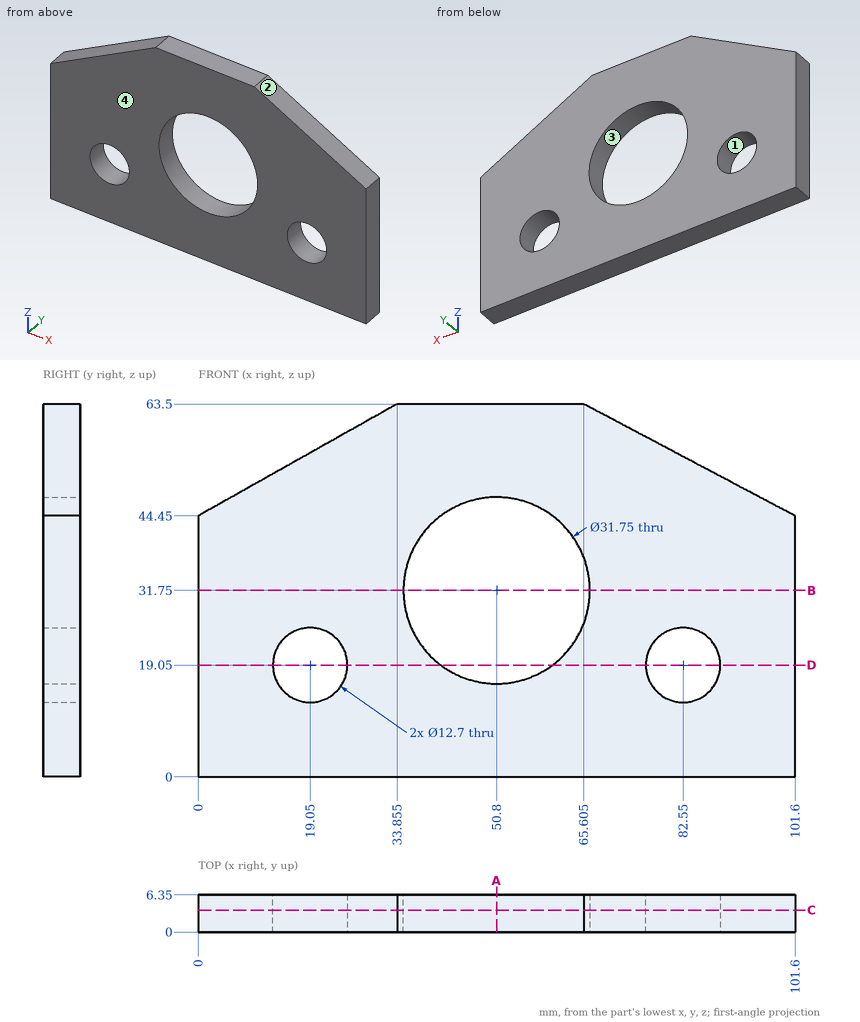
Verification items for this drawing (mm, ordinates from the low corner). Round coordinates to 2 decimals unless told otherwise and drop trailing zeros. Loops run counter-clockwise (first coordinate to the right, second up) from the corner with the lowest first, then second, coordinate; pieces in that order, holes last. Notation, with made-up numbers: (-34, 42) -> (-20, 42) arc R16 cw to (-20, 57) -> close; hole circle Ø4 at (79.25, 24). An arc over 180 degrees is marked (long way). Answer in a Markdown table with one row per item.
Q1. Sectioned sample at D-D on z = 19.05. Enter the section's corners in (x, y) (3 decimals), then the cut area to 3 significant figures.
Data:
| item | result |
|---|---|
| outline | (0, 0) -> (12.7, 0) -> (12.7, 6.35) -> (0, 6.35) -> close; (25.4, 0) -> (41.275, 0) -> (41.275, 6.35) -> (25.4, 6.35) -> close; (60.325, 0) -> (76.2, 0) -> (76.2, 6.35) -> (60.325, 6.35) -> close; (88.9, 0) -> (101.6, 0) -> (101.6, 6.35) -> (88.9, 6.35) -> close |
| area | 363 mm^2 |
Q2. Sectioned sample at B-B on z = 31.75. Enter the section's corners in (x, y) (3 decimals).
Data:
| item | result |
|---|---|
| outline | (0, 0) -> (34.925, 0) -> (34.925, 6.35) -> (0, 6.35) -> close; (66.675, 0) -> (101.6, 0) -> (101.6, 6.35) -> (66.675, 6.35) -> close |
Q3. Sectioned sample at A-A on x = 50.8. Enter the section's corners in (y, z) (3 decimals).
Data:
| item | result |
|---|---|
| outline | (0, 0) -> (6.35, 0) -> (6.35, 15.875) -> (0, 15.875) -> close; (0, 47.625) -> (6.35, 47.625) -> (6.35, 63.5) -> (0, 63.5) -> close |
Q4. Sectioned sample at C-C on y = 3.75. Enter the section's corners in (x, z) (3 decimals), then the cut area to 3 significant figures.
Data:
| item | result |
|---|---|
| outline | (0, 0) -> (101.6, 0) -> (101.6, 44.45) -> (65.605, 63.5) -> (33.855, 63.5) -> (0, 44.45) -> close; hole circle Ø12.7 at (19.05, 19.05); hole circle Ø31.75 at (50.8, 31.75); hole circle Ø12.7 at (82.55, 19.05) |
| area | 4,740 mm^2 |
Q5. Go/stop test with flat-tipped pins: P1, Ø3, axis at y = 1.5, z = 16, coming from the -X side; P2, Ø2, axis at x = 83, y = 3.5, coming from the +Z side. Record where each tip stops, or that it passes through.
Data:
| item | result |
|---|---|
| P1 | stops at x = 0 |
| P2 | stops at z = 54.82 |
Q6. Release check for a two-part mould opening along X. For the marked faces 1, 2, 3 and 4 record: released by +X, released by -X, zero draft, split by the parting line, or undercut.
Data:
| item | result |
|---|---|
| face 1 | undercut |
| face 2 | released by +X |
| face 3 | undercut |
| face 4 | zero draft |
Q7. Thickness scan on L1, parallel to Z at x = 50.8, y = 4.25 (3 decimals); L2, parallel to X at y = 4.5, z = 18.5; L3, parallel to X at y = 3.5, z = 32. Record the ranges inside material, lowest first.
Data:
| item | result |
|---|---|
| L1 | z = 0 to 15.875, 47.625 to 63.5 |
| L2 | x = 0 to 12.72, 25.38 to 42.06, 59.54 to 76.22, 88.88 to 101.6 |
| L3 | x = 0 to 34.93, 66.67 to 101.6 |
